Build history of the part. All positions in model axes, mm. A direction names the side the tool comes from. Round coordinates to 2 decimals unless told otherwise and drop trailing zeros. Write each loop counter-clockwise with the first axis right and the second up, starting at its lowest first coordinate (ties: lowest second). Pieces come first, ordered by that corner, then holes. Notation, with made-up numbers: M 26.5,-15.75 L 67.5,-15.75 A23 cw 67.5,18.25 Z; hole C 3,73.5 d3. An arc over 180 degrees is marked long. Use a Markdown table: item, result.
from build123d import *

# Parameters (mm, degrees)
SKETCH1_W           = 44
SKETCH1_H           = 29
SKETCH1_R           = 2.5
BOSS_EXTRUDE1_DEPTH = 30
CUT_EXTRUDE1_DEPTH  = 25
SKETCH3_W           = 20
SKETCH3_H           = 7
CUT_EXTRUDE2_DEPTH  = 29
SKETCH4_R           = 5
CUT_EXTRUDE3_DEPTH  = 3
THICKEN1_T1         = 2
CHAMFER1_SIZE       = 3
CHAMFER2_SIZE       = 4
CUT_EXTRUDE4_DEPTH  = 0.3


with BuildPart() as part:
    # Sketch1 → Boss-Extrude1 (new body)
    with BuildSketch(Plane.XY.offset(794.620141885)):
        with Locations((45.789156386, -208.298939869)):
            Rectangle(SKETCH1_W, SKETCH1_H)
        with Locations((52.789156386, -208.298939869)):
            Circle(SKETCH1_R, mode=Mode.SUBTRACT)
        with Locations((39.789156386, -208.298939869)):
            Circle(SKETCH1_R, mode=Mode.SUBTRACT)
    extrude(amount=BOSS_EXTRUDE1_DEPTH)

    # Sketch2 → Cut-Extrude1 (cut)
    with BuildSketch(Plane.XZ.offset(222.798939869)):
        Polygon((28.289156386, 816.620141885), (49.789156386, 816.620141885), (49.789156386, 806.620141885), (63.289156386, 806.620141885), (63.289156386, 796.620141885), (42.789156386, 796.620141885), (42.789156386, 806.620141885), (28.289156386, 806.620141885), align=None)
    extrude(amount=-CUT_EXTRUDE1_DEPTH, mode=Mode.SUBTRACT)

    # Sketch3 → Cut-Extrude2 (cut)
    with BuildSketch(Plane(origin=(42.789156386, 0, 0), x_dir=(0, 0, -1), z_dir=(1, 0, 0))):
        with Locations((-806.620141885, -201.298939869)):
            Rectangle(SKETCH3_W, SKETCH3_H)
    extrude(amount=CUT_EXTRUDE2_DEPTH, mode=Mode.SUBTRACT)

    # Sketch4 → Cut-Extrude3 (cut)
    with BuildSketch(Plane.XY.offset(824.620141885)):
        with Locations((39.789156386, -208.298939869)):
            Circle(SKETCH4_R)
        with Locations((52.789156386, -208.298939869)):
            Circle(SKETCH4_R)
    extrude(amount=-CUT_EXTRUDE3_DEPTH, mode=Mode.SUBTRACT)

    # Surface-Offset1: a surface, a copy of 1 face of the part
    surface_offset1_1 = part.part.faces().sort_by_distance((45.718963888, -208.298939869, 824.620141885))[0]
    add(Solid.thicken(surface_offset1_1, THICKEN1_T1))

    # Chamfer1
    chamfer1_edges = [part.edges().sort_by_distance(p)[0] for p in [
        (67.789156386, -222.798939869, 810.620141885),
        (23.789156386, -222.798939869, 810.620141885),
        (23.789156386, -193.798939869, 810.620141885),
        (67.789156386, -193.798939869, 810.620141885),
        (67.789156386, -208.298939869, 826.620141885),
        (45.789156386, -193.798939869, 826.620141885),
        (23.789156386, -208.298939869, 826.620141885),
        (45.789156386, -222.798939869, 826.620141885),
    ]]
    chamfer(chamfer1_edges, length=CHAMFER1_SIZE)

    # Chamfer2
    chamfer2_edges = [part.edges().sort_by_distance(p)[0] for p in [
        (42.789156386, -222.798939869, 801.620141885),
        (49.789156386, -222.798939869, 811.620141885),
    ]]
    chamfer(chamfer2_edges, length=CHAMFER2_SIZE)

    # Sketch5 → Cut-Extrude4 (cut)
    with BuildSketch(Plane.ZY.offset(-23.789156386)):
        with BuildLine():
            Line((818.620141885, -202.649682189), (818.620141885, -206.652086035))
            add(Edge.make_bspline(
                [(818.620141885, -206.652086035), (818.619252822, -206.919178198), (818.617545723, -207.432024737), (818.608027078, -208.166729139), (818.580745045, -208.834312551), (818.557267425, -209.434425918), (818.514456332, -209.967058232), (818.473538348, -210.433842751), (818.419974572, -210.832629594), (818.370229298, -211.074034458), (818.347705987, -211.183336035)],
                knots=[0, 0, 0, 0, 1.410062039, 2.707475311, 3.878576406, 4.937260626, 5.877586885, 6.699081471, 7.410979367, 8, 8, 8, 8], degree=3))
            add(Edge.make_bspline(
                [(818.347705987, -211.183336035), (818.311557144, -211.329662179), (818.240030609, -211.619192932), (818.088773389, -212.036013061), (817.914023625, -212.43337572), (817.707180436, -212.809789724), (817.471851613, -213.165289992), (817.206662217, -213.499344244), (816.910261737, -213.810042595), (816.590218995, -214.099775718), (816.243741522, -214.36240947), (815.875876555, -214.589684619), (815.488924875, -214.784299189), (815.081538972, -214.939665852), (814.657162625, -215.06465357), (814.212090229, -215.15281158), (813.748311447, -215.205673278), (813.431980786, -215.211055618), (813.271584192, -215.213784753)],
                knots=[0, 0, 0, 0, 1.02737288, 2.032829108, 3.019628684, 3.985738875, 4.958353778, 5.924249254, 6.890702889, 7.883913451, 8.865824512, 9.85161466, 10.829249435, 11.81541824, 12.821369441, 13.843154991, 14.906364023, 16, 16, 16, 16], degree=3))
            add(Edge.make_bspline(
                [(813.271584192, -215.213784753), (813.005097574, -215.205390696), (812.485113159, -215.189011716), (811.730483834, -215.036293795), (811.02652923, -214.786153381), (810.374229006, -214.441407876), (809.785954605, -214.002591168), (809.271001623, -213.47523327), (808.836100367, -212.862027363), (808.537719774, -212.288492765), (808.345728912, -211.781622), (808.209965299, -211.3631096), (808.106839718, -210.906236663), (808.013112973, -210.417557724), (807.941591938, -209.893298179), (807.89079841, -209.334513757), (807.858137784, -208.739806906), (807.853365927, -208.332151125), (807.850911115, -208.122438599)],
                knots=[0, 0, 0, 0, 1.260402266, 2.459371274, 3.627181936, 4.786749125, 5.93865593, 7.087644312, 8.261344208, 9.485713728, 10.136162886, 10.825977872, 11.566646758, 12.35154167, 13.181268117, 14.0701832, 15.007234106, 16, 16, 16, 16], degree=3))
            Line((807.850911115, -208.122438599), (798.620141885, -215.470195009))
            Line((798.620141885, -215.470195009), (798.620141885, -213.250643727))
            Line((798.620141885, -213.250643727), (807.850911115, -205.902887317))
            Line((807.850911115, -205.902887317), (807.850911115, -204.444553983))
            Line((807.850911115, -204.444553983), (798.620141885, -204.444553983))
            Line((798.620141885, -204.444553983), (798.620141885, -202.649682189))
            Line((798.620141885, -202.649682189), (818.620141885, -202.649682189))
        make_face()
        with BuildLine():
            Line((816.568859833, -204.444553983), (809.902193167, -204.444553983))
            Line((809.902193167, -204.444553983), (809.874148295, -208.106412958))
            add(Edge.make_bspline(
                [(809.874148295, -208.106412958), (809.874072657, -208.277384608), (809.87392605, -208.608776362), (809.896747622, -209.088208742), (809.922709465, -209.534609347), (809.962419927, -209.946270897), (810.013597756, -210.323376683), (810.077613908, -210.665740215), (810.152200057, -210.973913839), (810.26762556, -211.333350133), (810.45060064, -211.734593079), (810.716361518, -212.17119904), (811.052793662, -212.541742888), (811.431384321, -212.861223503), (811.85619796, -213.107304946), (812.308378702, -213.286409063), (812.784022722, -213.398806876), (813.110718973, -213.412169388), (813.275590603, -213.418912958)],
                knots=[0, 0, 0, 0, 1.14660753, 2.222451964, 3.218720504, 4.145691244, 4.995719623, 5.770487122, 6.480909919, 7.121111896, 8.299844659, 9.430703709, 10.534634535, 11.641396424, 12.741395289, 13.810956493, 14.895269934, 16, 16, 16, 16], degree=3))
            add(Edge.make_bspline(
                [(813.275590603, -213.418912958), (813.436472769, -213.412148659), (813.755282519, -213.398744286), (814.220730727, -213.286191288), (814.663169936, -213.104434652), (815.074166958, -212.849569783), (815.450349769, -212.541604679), (815.767772153, -212.175850326), (816.033594898, -211.77072656), (816.20222429, -211.391811004), (816.305816002, -211.053364398), (816.378622654, -210.759466647), (816.43761036, -210.426125104), (816.483472188, -210.054138637), (816.524742591, -209.644180232), (816.551501228, -209.195127342), (816.567674152, -208.707498527), (816.568455408, -208.369514628), (816.568859833, -208.194553983)],
                knots=[0, 0, 0, 0, 1.100801541, 2.181386982, 3.260112282, 4.364594493, 5.481957178, 6.577424609, 7.668452592, 8.790448866, 9.403819393, 10.091598921, 10.863153553, 11.720938239, 12.658472417, 13.685008818, 14.801622349, 16, 16, 16, 16], degree=3))
            Line((816.568859833, -208.194553983), (816.568859833, -204.444553983))
        make_face(mode=Mode.SUBTRACT)
    extrude(amount=-CUT_EXTRUDE4_DEPTH, mode=Mode.SUBTRACT)


solid = part.part
Q1. Two-plate mould, pull along X, no slides. Class faces 1 (the flat face through (53, -213, 796.62)), 2 (the flat face through (52, -197.799, 807)), 3 (the flat face through (67.789, -211, 809)): +X half, -X half, draft (parallel to the pull), parting line (faces both ways), or undercut.
Response values:
| item | result |
|---|---|
| face 1 | undercut |
| face 2 | draft |
| face 3 | +X half |
Q2. Cut at C-C on x = 40.5. Give the cut face in (y, z).
Response values:
| item | result |
|---|---|
| outline | M -222.8,794.62 L -210.7,794.62 L -210.7,806.62 L -221.09,806.62 L -221.09,796.62 L -222.8,796.62 Z; M -222.8,816.62 L -210.7,816.62 L -210.7,821.62 L -213.25,821.62 L -213.25,826.62 L -219.8,826.62 L -222.8,823.62 Z; M -205.9,794.62 L -193.8,794.62 L -193.8,823.62 L -196.8,826.62 L -203.35,826.62 L -203.35,821.62 L -205.9,821.62 L -205.9,816.62 L -197.8,816.62 L -197.8,806.62 L -205.9,806.62 Z |
Q3. Which spindle directions (+Z, -Z, +X, -X, +Y, -Y) get a long thin tool onto all of the face, cutting with end or side? Do faces 4 (the cylindrical face through (55.096, -212.735, 824.155)), 5 (the flat face through (43, -210, 816.62)), 6 (the flat face through (36, -210, 806.62)). Say none if no direction does.
Response values:
| item | result |
|---|---|
| face 4 | +Z |
| face 5 | none |
| face 6 | -Y |
Q4. Cut at B-B on z = 805. Give the cut face in (x, y), and give its area (3 significant figures).
Response values:
| item | result |
|---|---|
| outline | M 23.79,-219.8 L 26.79,-222.8 L 38.79,-222.8 L 42.79,-218.8 L 42.79,-197.8 L 67.79,-197.8 L 67.79,-196.8 L 64.79,-193.8 L 26.79,-193.8 L 23.79,-196.8 L 23.79,-202.65 L 24.09,-202.65 L 24.09,-204.44 L 23.79,-204.44 L 23.79,-208.17 L 24.09,-208.17 L 24.09,-210.39 L 23.79,-210.39 Z; M 63.29,-222.8 L 64.79,-222.8 L 67.79,-219.8 L 67.79,-204.8 L 63.29,-204.8 Z; hole C 39.79,-208.3 d5 |
| area | 685 mm2 |
Q5. Cut at D-D on x = 45.5. Give the cut face in (y, z).
Response values:
| item | result |
|---|---|
| outline | M -222.8,794.62 L -193.8,794.62 L -193.8,823.62 L -196.8,826.62 L -219.8,826.62 L -222.8,823.62 L -222.8,816.62 L -197.8,816.62 L -197.8,796.62 L -222.8,796.62 Z |
Q6. Cut at A-A on y = -216.75. Give the cut face in (x, z), and give its area (3 significant figures).
Response values:
| item | result |
|---|---|
| outline | M 23.79,794.62 L 67.79,794.62 L 67.79,823.62 L 64.79,826.62 L 26.79,826.62 L 23.79,823.62 Z; hole M 28.29,806.62 L 42.79,806.62 L 42.79,796.62 L 63.29,796.62 L 63.29,806.62 L 49.79,806.62 L 49.79,816.62 L 28.29,816.62 Z |
| area | 979 mm2 |
Q7. Drop flat-ended pins along their axis: P1, Ø4, axis at x = 52.79, y = -208.3, coming from the +Z side; P2, Ø8, axis at x = 52.79, y = -208.3, coming from the +Z side; P3, Ø5, axis at x = 50, z = 812, coming from the -Y side. Give the stop position or say it passes through.
Response values:
| item | result |
|---|---|
| P1 | passes through |
| P2 | stops at z = 821.62 |
| P3 | stops at y = -221.51 |
Q8. Drill centre lines: L1, parallel to X at y = -208.5, z = 804; L2, parallel to Z at x = 43, y = -200; L3, parallel to X at y = -217.5, z = 798. Where is each one in solid material? Low to high.
Response values:
| item | result |
|---|---|
| L1 | x = 23.79 to 37.3, 42.28 to 42.79, 63.29 to 67.79 |
| L2 | z = 794.62 to 796.62, 816.62 to 826.62 |
| L3 | x = 23.79 to 42.79, 63.29 to 67.79 |
